```python
from build123d import *

# Parameters (mm, degrees)
SKETCH2_W           = 80
SKETCH2_H           = 20
BOSS_EXTRUDE1_DEPTH = 5
FILLET1_R           = 5
SHELL1_T            = -2
SKETCH3_W           = 6
SKETCH3_H           = 5
BOSS_EXTRUDE2_DEPTH = 6
SKETCH4_R           = 1.425
CUT_EXTRUDE1_DEPTH  = 4


with BuildPart() as part:
    # Sketch2 → Boss-Extrude1 (new body)
    with BuildSketch(Plane.XY):
        Rectangle(SKETCH2_W, SKETCH2_H)
    extrude(amount=BOSS_EXTRUDE1_DEPTH)

    # Fillet1
    fillet1_edges = [part.edges().sort_by_distance(p)[0] for p in [
        (-40, 10, 2.5),
        (40, 10, 2.5),
        (40, -10, 2.5),
        (-40, -10, 2.5),
    ]]
    fillet(fillet1_edges, radius=FILLET1_R)

    # Shell1
    shell1_openings = [part.faces().sort_by_distance(p)[0] for p in [
        (0, 0, 5),
    ]]
    offset(amount=SHELL1_T, openings=shell1_openings, kind=Kind.INTERSECTION)

    # Sketch3 → Boss-Extrude2 (add)
    with BuildSketch(Plane.XZ.offset(10)):
        with Locations((0, 2.5)):
            Rectangle(SKETCH3_W, SKETCH3_H)
    extrude(amount=BOSS_EXTRUDE2_DEPTH)

    # Sketch4 → Cut-Extrude1 (cut)
    with BuildSketch(Plane.XZ.offset(16)):
        with Locations((0, 2.5)):
            Circle(SKETCH4_R)
    extrude(amount=-CUT_EXTRUDE1_DEPTH, mode=Mode.SUBTRACT)


solid = part.part
```
For this review, take the finished solid that the model builds, in its own axes (mm). A direction names the side the tool comes from. Give positions to 0.01 mm unless a question says otherwise; leave off trailing zeros. Order: outer loops, then holes, each group sorted by start corner. A loop starts at its lowest first (then second) coordinate and runs counter-clockwise, first axis right, second up.
1) Take a section at D-D (y = -11). Give the boundary of the cut face in (x, z).
2) Take a section at A-A (x = -26). Give the boundary of the cut face in (y, z), then the cut area to 3 significant figures.
3) Wall thickness on line 1 (X direction, y = -12.25, z = 2.7); line 2 (X direction, y = 4.5, z = 2.7); line 3 (Y direction, x = 11.5, z = 4): over which ranges is each line inside the solid? List them lowest first.
4) Insertion check: pin 1 (2 mm diameter, centred on x = -13, z = 2, fed in from -Y); pin 2 (1.5 mm diameter, centred on y = -11, z = 2.5, fed in from +X); pin 3 (1.5 mm diameter, centred on x = -22.5, y = 7, fed in from +Z). Each pin has a flat end and moves straight along its axis. Give the tip position at first contact, or say it passes through.
5) The part is to be moulded in two halves that separate along Y. For faces 6 (the face through (0, 10, 2)), 7 (the face through (0, -16, 4.2)), 8 (the face through (-37.14, -7.1, 3.52)), 9 (the face through (0, 8, 3)), say which applies: released by +Y, released by -Y, zero draft, split by the parting line, or undercut.
6) For faces 1 (the face through (37.14, 7.1, 3.52)), 2 (the face through (40, 0, 2)), 3 (the face through (19, -10, 2)), 4 (the face through (0, -9, 5)), 5 (the face through (-3, -13, 2)), list the 3-axis set-ups (+Z, -Z, +X, -X, +Y, -Y) from which the entire face can be reached by the end or side of a thin tool; tool diameter is ignored.
7) Take a section at C-C (x = 0). Give the boundary of the cut face in (y, z) (3 decimals), then the cut area to 3 significant figures.
8) Take a section at B-B (y = -3.5). Give the boundary of the cut face in (x, z), then the cut area to 3 significant figures.
Derived:
1. outline: (-3, 0) - (3, 0) - (3, 5) - (-3, 5) - close
2. outline: (-10, 0) - (10, 0) - (10, 5) - (8, 5) - (8, 2) - (-8, 2) - (-8, 5) - (-10, 5) - close
2. area: 52.0 mm2
3. line 1: x = -3 to -1.41, 1.41 to 3
3. line 2: x = -40 to -38, 38 to 40
3. line 3: y = -10 to -8, 8 to 10
4. pin 1: stops at y = -10
4. pin 2: stops at x = 3
4. pin 3: stops at z = 2
5. face 6: released by +Y
5. face 7: released by -Y
5. face 8: undercut
5. face 9: undercut
6. face 1: +Z
6. face 2: +Z, -Z, +X, +Y, -Y
6. face 3: +Z, -Z, +X, -Y
6. face 4: +Z, +X, -X, +Y, -Y
6. face 5: +Z, -Z, -X, -Y
7. outline: (-16, 0) - (10, 0) - (10, 5) - (8, 5) - (8, 2) - (-8, 2) - (-8, 5) - (-16, 5) - (-16, 3.925) - (-12, 3.925) - (-12, 1.075) - (-16, 1.075) - close
7. area: 70.6 mm2
8. outline: (-40, 0) - (40, 0) - (40, 5) - (38, 5) - (38, 2) - (-38, 2) - (-38, 5) - (-40, 5) - close
8. area: 172 mm2
